Work out the finished part from the listing and answer in its coordinate system (mm). A direction names the side the tool comes from. Round coordinates to 2 decimals unless told otherwise and drop trailing zeros. Write each loop counter-clockwise with the first axis right and the second up, starting at its lowest first coordinate (ties: lowest second). Pieces come first, ordered by that corner, then holes. Notation, with made-up numbers: M 34,22 L 45,22 A28 ccw 45,44 Z; hole C 40,72.5 d7. An arc over 180 degrees is marked long. Answer in a Markdown table with one row per item.
```python
from build123d import *

# Parameters (mm, degrees)
BOSS_EXTRUDE1_DEPTH = 15.75
CUT_EXTRUDE1_DEPTH  = 29.12540638


with BuildPart() as part:
    # Sketch1 → Boss-Extrude1 (new body)
    with BuildSketch(Plane(origin=(-15.864839006, 0, -9.159569071), x_dir=(0.5, 0, -0.866025404), z_dir=(0.866025404, 0, 0.5))):
        Polygon((-250.897888289, -141.485825414), (-306.1863183, -164.792251717), (-304.632556546, -168.478147051), (-249.344126536, -145.171720748), align=None)
    extrude(amount=-BOSS_EXTRUDE1_DEPTH)

    # Sketch2 → Cut-Extrude1 (cut, through all)
    with BuildSketch(Plane(origin=(6.393069309, -30.331785785, -11.073120859), x_dir=(0.980957953, 0.182442937, 0.066603816), z_dir=(-0.194220219, 0.921473834, 0.336399287))):
        Polygon((-192.659600657, -289.596321832), (-189.22286398, -291.424710992), (-165.922780405, -248.036843291), (-175.386750656, -243.001886517), (-198.517574459, -286.479802644), align=None)
        Polygon((-149.766129503, -256.632394287), (-172.896953306, -300.110310414), (-178.754927107, -296.993791227), (-182.191663785, -295.165402067), (-159.230099754, -251.597437512), align=None)
    extrude(amount=-CUT_EXTRUDE1_DEPTH, mode=Mode.SUBTRACT)


solid = part.part
```
1. A tool of negligible diameter and unlimited length cuts with its end or side. For faces 4 (the flat face through (-147.678, -147.479, 215.006)), 5 (the flat face through (-158.21, -154.4, 221.85)), from which of +Z, -Z, +X, -X, +Y, -Y can it reach the whole face along a straight path? Write none if from no direction.
Calculated:
| item | result |
|---|---|
| face 4 | +Z, -Y |
| face 5 | -Z, +X, -Y |
2. The part is cut by section B-B (x = -173). Determine the outline of the cut face in (y, z), plus the area to 3 significant figures.
Calculated:
| item | result |
|---|---|
| outline | M -168.48,251.88 L -163.92,239.38 L -159.58,239.4 L -164.79,253.67 Z |
| area | 58.1 mm² |
3. The part is cut by section A-A (y = -147.25). Determine the outline of the cut face in (x, z).
Calculated:
| item | result |
|---|---|
| outline | M -159.57,208.25 L -156.64,203.17 L -143,211.05 L -145.93,216.13 L -149.47,214.08 L -151.67,217.93 L -158.27,214.13 L -156.04,210.29 Z |
4. Consider line 1 along Y through (x, z) = (-159.5, 230.5); line 2 along X through (y, z) = (-163.25, 243.5); line 3 along Y through (x, z) = (-160, 226). Determine where each line is inside the solid, lowest interval first. Write a range as from..to.
Calculated:
| item | result |
|---|---|
| line 1 | y = -157.83..-153.49 |
| line 2 | x = -175.4..-166.29 |
| line 3 | y = -156.29..-151.95 |
5. The part is cut by section C-C (z = 223). Determine the outline of the cut face in (x, y).
Calculated:
| item | result |
|---|---|
| outline | M -163.45,-155.92 L -154.56,-154.05 L -154.57,-149.71 L -163.44,-151.58 Z |
6. Determine the mould class of faces 1 (the flat face through (-157.73, -147.48, 209.2)), 2 (the flat face through (-147.644, -143.355, 203.56)), 3 (the flat face through (-158.6, -150.39, 222.53)) for opening direction Z: released by +Z, released by -Z, zero draft, split by the parting line, or undercut.
Calculated:
| item | result |
|---|---|
| face 1 | undercut |
| face 2 | released by -Z |
| face 3 | released by +Z |
7. Given pin 1 (10 mm diameter, centred on x = -172, y = -158, fed in from -Z); pin 2 (8 mm diameter, centred on x = -162, z = 229, fed in from -Y); pin 3 (2 mm diameter, centred on y = -160, z = 236, fed in from +X), each flat-ended and moving along its own axis, determine where each tip first touches the part or whether it passes through.
Calculated:
| item | result |
|---|---|
| pin 1 | stops at z = 229.09 |
| pin 2 | stops at y = -159.49 |
| pin 3 | stops at x = -161.43 |
